```python
from build123d import *

# Parameters (mm, degrees)
BOSS_EXTRUDE1_DEPTH     = 50
BOSS_EXTRUDE2_DEPTH     = 10
BOSS_EXTRUDE3_DEPTH     = 4
SKETCH3_W               = 40
SKETCH3_H               = 30.268164841
CUT_EXTRUDE1_DEPTH      = 36
CUT_EXTRUDE1_DEPTH_BACK = 36


with BuildPart() as part:
    # Sketch2 → Boss-Extrude1 (new body, symmetric)
    with BuildSketch(Plane(origin=(0, 0, 0), x_dir=(0, 0, -1), z_dir=(1, 0, 0))):
        Polygon((-35, 0), (35, 0), (10, 50), (-10, 50), align=None)
    extrude(amount=BOSS_EXTRUDE1_DEPTH, both=True)

    # Sketch2<5> → Boss-Extrude2 (add, symmetric)
    with BuildSketch(Plane(origin=(0, 0, 0), x_dir=(0, 0, -1), z_dir=(1, 0, 0))):
        with BuildLine():
            ThreePointArc((19.865917579, 30.268164841), (0, 78), (-19.865917579, 30.268164841))
            Line((-19.865917579, 30.268164841), (-17.959919678, 34.080160643))
            ThreePointArc((-17.959919678, 34.080160643), (0, 74), (17.959919678, 34.080160643))
            Line((17.959919678, 34.080160643), (19.865917579, 30.268164841))
        make_face()
    extrude(amount=BOSS_EXTRUDE2_DEPTH, both=True)

    # Sketch2<6> → Boss-Extrude3 (add, symmetric)
    with BuildSketch(Plane(origin=(0, 0, 0), x_dir=(0, 0, -1), z_dir=(1, 0, 0))):
        Polygon((-35, 0), (35, 0), (10, 50), (-10, 50), align=None)
        with BuildLine():
            Line((-19.865917579, 30.268164841), (19.865917579, 30.268164841))
            ThreePointArc((19.865917579, 30.268164841), (0, 78), (-19.865917579, 30.268164841))
        make_face()
    extrude(amount=BOSS_EXTRUDE3_DEPTH, both=True)

    # Sketch3 → Cut-Extrude1 (cut, two sides)
    with BuildSketch(Plane.XY) as cut_extrude1_sk:
        Polygon((38, 15), (50, 15), (50, 50), (18.5, 50), align=None)
        with Locations((0, 15.134082421)):
            Rectangle(SKETCH3_W, SKETCH3_H)
        Polygon((-38, 15), (-18.5, 50), (-50, 50), (-50, 15), align=None)
    extrude(amount=CUT_EXTRUDE1_DEPTH, mode=Mode.SUBTRACT)
    extrude(cut_extrude1_sk.sketch, amount=-CUT_EXTRUDE1_DEPTH_BACK, mode=Mode.SUBTRACT)


solid = part.part
```
Check sheet for the modelled part. Datum: model origin and axes. Units: mm. A direction names the side the tool comes from. Round coordinates to 2 decimals unless told otherwise and drop trailing zeros. Order: outer loops, then holes, each group sorted by start corner. A loop starts at its lowest first (then second) coordinate and runs counter-clockwise, first axis right, second up. Notation, with made-up numbers: (-23, -31) -> (0, -31) arc R22 cw to (0, -1) -> close; hole circle Ø11 at (2.5, 72). An arc over 180 degrees is marked (long way). One line per item, written item: value. Start each with the question number.
Q1. Cross-section at D-D (x = 7). Record the boundary of the cut face in (y, z), and give its area (3 significant figures).
Q2. Thickness scan on line 1 (X direction, y = 9.5, z = -22.5); line 2 (Y direction, x = 15, z = 16); line 3 (X direction, y = 29.5, z = 11.5). Record the ranges inside material, lowest first.
Q3. Cross-section at A-A (z = 22.5). Record the boundary of the cut face in (x, y).
Q4. Mould release check, pull along Z, two halves, no side actions. Record for faces 1 (the face through (-11, 50, 0)), 2 (the face through (10, 74, 4)), 3 (the face through (0.14, 77.985, -0.922)): pulls with the +Z half, pulls with the -Z half, needs draft (parallel to the pull), parting line crosses it, or undercut.
Q5. Set-up check for faces 4 (the face through (44, 15, 0)), 5 (the face through (20, 15, 0)), 6 (the face through (-4, 59, 0)), 7 (the face through (-44, 15, 0)), 8 (the face through (4, 59, 0)): record each of +Z, -Z, +X, -X, +Y, -Y from which the full face is reachable in a straight line by a thin tool's end or side.
Q6. Gauge pin test, flat ends, axial feed: pin 1 Ø4.5 at (x, z) = (10, 0.5) entering from +Y; pin 2 Ø10 at (x, y) = (24, 19) entering from +Z; pin 3 Ø1 at (x, z) = (-2, -15) entering from +Y. Record the tip position at first contact, or that the pin passes through.
Q7. Cross-section at C-C (y = 23.5). Record the boundary of the cut face in (x, z), and give its area (3 significant figures).
Q8. Cross-section at B-B (z = 0). Record the boundary of the cut face in (x, y).
Completed:
1. outline: (30.27, -19.87) arc R28 ccw (long way) to (30.27, 19.87) -> close; hole (34.08, -17.96) arc R24 ccw (long way) to (34.08, 17.96) -> (50, 10) -> (50, -10) -> close
1. area: 1,070 mm²
2. line 1: x = -50 to -20, 20 to 50
2. line 2: y = 30.27 to 38
2. line 3: x = -29.92 to -20, 20 to 29.92
3. outline: (-50, 0) -> (-20, 0) -> (-20, 25) -> (-32.43, 25) -> (-38, 15) -> (-50, 15) -> close; (-10, 33.33) -> (10, 33.33) -> (10, 41.65) -> (4, 41.65) -> (4, 58.35) -> (10, 58.35) -> (10, 66.67) -> (-10, 66.67) -> (-10, 58.35) -> (-4, 58.35) -> (-4, 41.65) -> (-10, 41.65) -> close; (20, 0) -> (50, 0) -> (50, 15) -> (38, 15) -> (32.43, 25) -> (20, 25) -> close
4. face 1: undercut
4. face 2: needs draft
4. face 3: parting line crosses it
5. face 4: +Z, -Z, +X, +Y
5. face 5: +Z, -Z, -Y
5. face 6: -X
5. face 7: +Z, -Z, -X, +Y
5. face 8: +X
6. pin 1: stops at y = 78
6. pin 2: stops at z = 28
6. pin 3: stops at y = 73.95
7. outline: (-33.26, -23.25) -> (-20, -23.25) -> (-20, 23.25) -> (-33.26, 23.25) -> close; (20, -23.25) -> (33.26, -23.25) -> (33.26, 23.25) -> (20, 23.25) -> close
7. area: 1,230 mm²
8. outline: (-50, 0) -> (-20, 0) -> (-20, 30.27) -> (20, 30.27) -> (20, 0) -> (50, 0) -> (50, 15) -> (38, 15) -> (18.5, 50) -> (4, 50) -> (4, 74) -> (10, 74) -> (10, 78) -> (-10, 78) -> (-10, 74) -> (-4, 74) -> (-4, 50) -> (-18.5, 50) -> (-38, 15) -> (-50, 15) -> close
